Solid Edge part; units mm, degrees
sketch "Sketch1" plane through (0, 0, 0) normal (0, 0, 1) x (1, 0, 0)
  line L0 (-225, -85) -> (225, -85)
  line L1 (225, -85) -> (225, 85)
  line L2 (225, 85) -> (-225, 85)
  line L3 (-225, 85) -> (-225, -85)
  dimension "D1" = 225
  dimension "D2" = 225
extrude "Protrusion1" add sketch "Sketch1" along normal blind 3
sketch "Sketch2" plane through (0, 0, 3) normal (0, 0, 1) x (1, 0, 0)
  circle A0 centre (-190, 57.5) radius 3
  circle A1 centre (-190, -57.5) radius 3
  circle A2 centre (190, -57.5) radius 3
  circle A3 centre (190, 57.5) radius 3
  dimension "D1" = 190
  dimension "D2" = 190
extrude "Cutout1" cut sketch "Sketch2" against normal through all
sketch "Sketch3" plane through (0, 0, 3) normal (0, 0, 1) x (1, 0, 0)
  circle A0 centre (-15.5, 15.5) radius 2
  circle A1 centre (15.5, 15.5) radius 2
  circle A2 centre (15.5, -15.5) radius 2
  circle A3 centre (-15.5, -15.5) radius 2
  dimension "D1" = 15.5
extrude "Cutout2" cut sketch "Sketch3" against normal through all
sketch "Sketch4" plane through (-112.5, 0, 3) normal (0, 0, 1) x (1, 0, 0)
  circle A0 centre (-12.5, -57.5) radius 3
  dimension "D1" = 12.5
extrude "Cutout3" cut sketch "Sketch4" against normal through all
sketch "Sketch5" plane through (-112.5, 0, 3) normal (0, 0, 1) x (1, 0, 0)
  line L0 (112.5, 85) -> (-52.5, 85)
  line L1 (-52.5, 85) -> (-52.5, -35)
  line L2 (-52.5, -35) -> (112.5, -35)
  line L3 (112.5, -35) -> (112.5, 85)
  dimension "D1" = 52.5
  dimension "D2" = 52.5
extrude "Extrusionsausprägung_2" add sketch "Sketch5" along normal blind 3
sketch "Sketch6" plane through (-112.5, 0, 3) normal (0, 0, 1) x (1, 0, 0)
  circle A0 centre (72.5, 57.5) radius 3
  circle A1 centre (72.5, -57.5) radius 3
extrude "Cutout4" cut sketch "Sketch6" against normal through all
sketch "Sketch7" plane through (-112.5, 0, 0) normal (0, 0, -1) x (1, 0, 0)
  circle A0 centre (72.5, -57.5) radius 3
  circle A1 centre (97, 15.5) radius 2
  circle A2 centre (97, -15.5) radius 2
extrude "Cutout5" cut sketch "Sketch7" against normal through all
mirror "Mirror1" about plane through (0, 0, 0) normal (1, 0, 0) of "Extrusionsausprägung_2", "Cutout3"
mirror "Mirror2" about plane through (0, 0, 0) normal (1, 0, 0) of "Extrusionsausprägung_2", "Cutout3", "Cutout1"
mirror "Mirror3" about plane through (0, 0, 0) normal (1, 0, 0) of "Cutout5", "Cutout4"
sketch "Sketch8" plane through (0, 25, 6) normal (0, 0, 1) x (1, 0, 0)
  line L0 (0, 60) -> (0, -110)
extrude "Cutout8" cut sketch "Sketch8" against normal through all material side at (-0.05, 0, 6)
sketch "Sketch9" plane through (112.5, 0, 0) normal (0, 0, -1) x (1, 0, 0)
  circle A0 centre (-112.5, 0) radius 11
extrude "Cutout9" cut sketch "Sketch9" against normal through all
properties material "Nylon, allgemein"
Could you check a few things on this model? Use its own coordinates, in mm. A direction names the side the tool comes from. Coordinates: 2 decimals unless noted, no trailing zeros. Write each loop counter-clockwise with the first axis right and the second up, starting at its lowest first coordinate (ties: lowest second). Pieces come first, ordered by that corner, then holes. Notation, with made-up numbers: (-7.5, 1.5) - (13.5, 1.5) arc R15 ccw to (13.5, 20.5) - close; hole circle Ø9 at (48, 78). An arc over 180 degrees is marked (long way). Use a Markdown table: item, result.
Q1. Please list where these lines run through material, in increasing order: L1, parallel to Y at x = 190, z = 2.35; L2, parallel to X at y = 57.5, z = 0.6; L3, parallel to Y at x = 15.5, z = 4.9.
Geometry check:
| item | result |
|---|---|
| L1 | y = -85 to -60.5, -54.5 to 54.5, 60.5 to 85 |
| L2 | x = 0 to 37, 43 to 187, 193 to 225 |
| L3 | y = -35 to -17.5, -13.5 to 13.5, 17.5 to 85 |
Q2. Imagine slicing it at C-C (z = 4). List the corners of the cut face in (x, y) for me, and give its area (3 significant figures).
Geometry check:
| item | result |
|---|---|
| outline | (0, -35) - (165, -35) - (165, 85) - (0, 85) - (0, 11) arc R11 cw to (0, -11) - close; hole circle Ø4 at (15.5, -15.5); hole circle Ø4 at (15.5, 15.5); hole circle Ø6 at (40, 57.5) |
| area | 19,600 mm2 |
Q3. Imagine slicing it at B-B (x = 125). List the corners of the cut face in (y, z) for me, and give its area (3 significant figures).
Geometry check:
| item | result |
|---|---|
| outline | (-85, 0) - (-60.5, 0) - (-60.5, 3) - (-85, 3) - close; (-54.5, 0) - (85, 0) - (85, 6) - (-35, 6) - (-35, 3) - (-54.5, 3) - close |
| area | 852 mm2 |
Q4. Thinking about a two-plate mould opening in Y: for faces 3 (the cylindrical face through (42.21, -59.53, 1.52)), 4 (the cylindrical face through (11, 0, 3)), 5 (the flat face through (81, 26, 6)), 6 (the flat face through (114, 85, 3)), which applies, +Y half, -Y half, draft (parallel to the pull), parting line (faces both ways), or undercut?
Geometry check:
| item | result |
|---|---|
| face 3 | undercut |
| face 4 | undercut |
| face 5 | draft |
| face 6 | +Y half |
Q5. Imagine slicing it at A-A (y = -57.5). List the corners of the cut face in (x, z) for me.
Geometry check:
| item | result |
|---|---|
| outline | (0, 0) - (37, 0) - (37, 3) - (0, 3) - close; (43, 0) - (122, 0) - (122, 3) - (43, 3) - close; (128, 0) - (187, 0) - (187, 3) - (128, 3) - close; (193, 0) - (225, 0) - (225, 3) - (193, 3) - close |
Q6. I'm going to push flat-ended pins straight in: pin 1 Ø1 at (x, z) = (102, 4.5) entering from -Y; pin 2 Ø3.5 at (x, y) = (40, 57.5) entering from +Z; pin 3 Ø9.5 at (x, y) = (190, -57.5) entering from +Z. Where does each tip first touch, or does it pass through?
Geometry check:
| item | result |
|---|---|
| pin 1 | stops at y = -35 |
| pin 2 | passes through |
| pin 3 | stops at z = 3 |
Q7. Which directions (+Z, -Z, +X, -X, +Y, -Y) give clear straight access to the entire face, cutting with the end or side of a thin tool? Please do faces 1 (the flat face through (136, -37, 3)), 2 (the cylindrical face through (42.21, 59.53, 2.96)).
Geometry check:
| item | result |
|---|---|
| face 1 | +Z, +X, -Y |
| face 2 | +Z, -Z |
Q8. Imagine slicing it at D-D (y = 47). List the corners of the cut face in (x, z) for me, and give its area (3 significant figures).
Geometry check:
| item | result |
|---|---|
| outline | (0, 0) - (225, 0) - (225, 3) - (165, 3) - (165, 6) - (0, 6) - close |
| area | 1,170 mm2 |
